The listing builds one solid part. Answer for the finished solid, in the listing's coordinates (mm). A direction names the side the tool comes from. Give positions to 0.01 mm unless a question says otherwise; leave off trailing zeros. Order: outer loops, then holes, each group sorted by start corner. A loop starts at its lowest first (then second) coordinate and runs counter-clockwise, first axis right, second up. Notation, with made-up numbers: (-30, -17) -> (17, -17) arc R10 ccw to (17, -11) -> close; hole circle Ø4 at (60, 55). An arc over 180 degrees is marked (long way). One line per question, with ' | ' between items. Start each with the question number.
```python
from build123d import *

# Parameters (mm, degrees)
F1_DEPTH      = 15
F1_DEPTH_BACK = 15
F2_R          = 2
F3_DEPTH      = 5
F3_DEPTH_BACK = 5
F4_R          = 2
F5_DEPTH      = 5
F5_DEPTH_BACK = 5


with BuildPart() as f1:
    # F0 (on Front) → F1 (new body, two sides)
    with BuildSketch(Plane.XZ) as f1_sk:
        Polygon((10, -10), (-10, -10), (-10, -13), (13, -13), (13, 7), (58.1, 7), (58.1, 33.5), (22.55, 33.5), (22.55, 30.5), (55.1, 30.5), (55.1, 10), (10, 10), align=None)
    extrude(amount=F1_DEPTH)
    extrude(f1_sk.sketch, amount=-F1_DEPTH_BACK)

    # F2 (on face) → F3 (cut, two sides)
    with BuildSketch(Plane.YZ.offset(13)) as f3_sk:
        Circle(F2_R)
    extrude(amount=-F3_DEPTH, mode=Mode.SUBTRACT)
    extrude(f3_sk.sketch, amount=-F3_DEPTH_BACK, mode=Mode.SUBTRACT)

    # F4 (on face) → F5 (cut, two sides)
    with BuildSketch(Plane(origin=(0, 0, -13), x_dir=(1, 0, 0), z_dir=(0, 0, -1))) as f5_sk:
        Circle(F4_R)
    extrude(amount=-F5_DEPTH, mode=Mode.SUBTRACT)
    extrude(f5_sk.sketch, amount=-F5_DEPTH_BACK, mode=Mode.SUBTRACT)


solid = f1.part
```
(1) The part is cut by section D-D on y = -3.5. Determine the outline of the cut face in (x, z).
(2) Given P1, Ø1, axis at x = -3, y = 5, coming from the +Z side; P2, Ø9, axis at x = 28, y = -1, coming from the -Z side; P3, Ø6, axis at y = -2.5, z = -8, coming from the +X side, each flat-ended and moving along its own axis, determine where each tip first touches the part or whether it passes through.
(3) Determine the mould class of faces 6 (the face through (55.1, 0, 20)), 7 (the face through (10, -0.2, 2.4)), 8 (the face through (35, 0, 7)) for opening direction Z: pulls with the +Z half, pulls with the -Z half, needs draft (parallel to the pull), parting line crosses it, or undercut.
(4) The part is cut by section C-C on y = 0. Determine the outline of the cut face in (x, z), plus the area to 3 significant figures.
(5) Consider line 1 (Z direction, x = 35.5, y = -3.75); line 2 (Y direction, x = 0, z = -11); line 3 (X direction, y = 0, z = -11.55). Determine where each line is inside the solid, lowest interval first.
(6) The part is cut by section B-B on z = 0. Determine the outline of the cut face in (x, y), plus the area to 3 significant figures.
(7) For faces 1 (the face through (13, 0, -3)), 2 (the face through (58.1, 0, 20)), 3 (the face through (29, -15, 9)), 4 (the face through (33, 0, 10)), 5 (the face through (2.4, -0.2, -10)), determine the directions among +Z, -Z, +X, -X, +Y, -Y from which every point of the face is accessible in a straight line to the end or side of a thin tool.
(8) The part is cut by section A-A on x = 33.5. Determine the outline of the cut face in (y, z), plus the area to 3 significant figures.
Result sheet:
1) outline: (-10, -13) -> (13, -13) -> (13, 7) -> (58.1, 7) -> (58.1, 33.5) -> (22.55, 33.5) -> (22.55, 30.5) -> (55.1, 30.5) -> (55.1, 10) -> (10, 10) -> (10, -10) -> (-10, -10) -> close
2) P1: stops at z = -10 | P2: stops at z = 7 | P3: stops at x = 13
3) face 6: undercut | face 7: needs draft | face 8: pulls with the -Z half
4) outline: (-10, -13) -> (-2, -13) -> (-2, -10) -> (-10, -10) -> close; (2, -13) -> (13, -13) -> (13, -2) -> (10, -2) -> (10, -10) -> (2, -10) -> close; (10, 2) -> (13, 2) -> (13, 7) -> (58.1, 7) -> (58.1, 33.5) -> (22.55, 33.5) -> (22.55, 30.5) -> (55.1, 30.5) -> (55.1, 10) -> (10, 10) -> close | area: 408 mm^2
5) line 1: z = 7 to 10, 30.5 to 33.5 | line 2: y = -15 to -2, 2 to 15 | line 3: x = -10 to -2, 2 to 13
6) outline: (10, -15) -> (13, -15) -> (13, -2) -> (10, -2) -> close; (10, 2) -> (13, 2) -> (13, 15) -> (10, 15) -> close | area: 78.0 mm^2
7) face 1: -Z, +X, +Y, -Y | face 2: +Z, -Z, +X, +Y, -Y | face 3: +Z, -Z, +X, -X, -Y | face 4: -X, +Y, -Y | face 5: +Z, -X, +Y, -Y
8) outline: (-15, 7) -> (15, 7) -> (15, 10) -> (-15, 10) -> close; (-15, 30.5) -> (15, 30.5) -> (15, 33.5) -> (-15, 33.5) -> close | area: 180 mm^2
